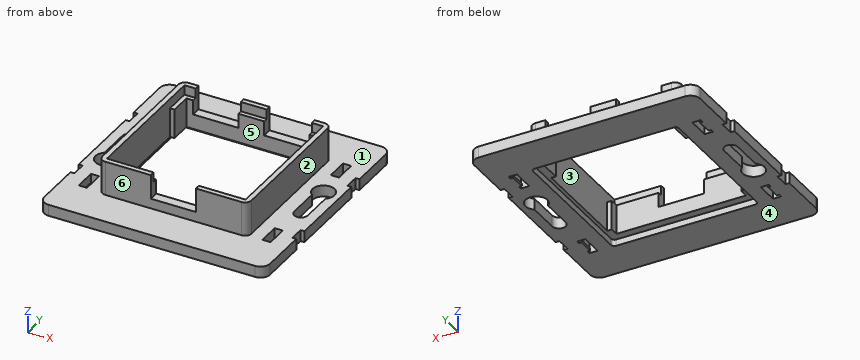
```python
from build123d import *

# Parameters (mm, degrees)
F0_W      = 40.2
F0_H      = 40.2
F1_DEPTH  = 14.1
F2_DEPTH  = 3.5
F3_W      = 1.2
F3_H      = 4.5
F4_DEPTH  = 25
F6_DEPTH  = 2
F7_W      = 43
F7_H      = 43
F7_W_2    = 40.2
F7_H_2    = 40.2
F8_DEPTH  = 3
F9_W      = 14
F9_H      = 7.5
F10_DEPTH = 5
F11_W     = 14
F11_H     = 7.5
F12_DEPTH = 5
F13_W     = 1.4
F13_H     = 31
F14_DEPTH = 15
F15_W     = 0.8
F15_H     = 4.8
F16_DEPTH = 2.7
F17_DEPTH = 7


with BuildPart() as f1:
    # F0 (on Top) → F1 (new body)
    with BuildSketch(Plane.XY):
        with BuildLine():
            Line((23.1, -21.1), (23.1, 21.1))
            ThreePointArc((23.1, 21.1), (22.514214, 22.514214), (21.1, 23.1))
            Line((21.1, 23.1), (-21.1, 23.1))
            ThreePointArc((-21.1, 23.1), (-22.514214, 22.514214), (-23.1, 21.1))
            Line((-23.1, 21.1), (-23.1, -21.1))
            ThreePointArc((-23.1, -21.1), (-22.514214, -22.514214), (-21.1, -23.1))
            Line((-21.1, -23.1), (21.1, -23.1))
            ThreePointArc((21.1, -23.1), (22.514214, -22.514214), (23.1, -21.1))
        make_face()
        Rectangle(F0_W, F0_H, mode=Mode.SUBTRACT)
    extrude(amount=F1_DEPTH)

    # F0 (on Top) → F2 (join)
    with BuildSketch(Plane.XY):
        with BuildLine():
            Line((32, 35), (-32, 35))
            ThreePointArc((-32, 35), (-34.12132, 34.12132), (-35, 32))
            Line((-35, 32), (-35, -32))
            ThreePointArc((-35, -32), (-34.12132, -34.12132), (-32, -35))
            Line((-32, -35), (32, -35))
            ThreePointArc((32, -35), (34.12132, -34.12132), (35, -32))
            Line((35, -32), (35, 32))
            ThreePointArc((35, 32), (34.12132, 34.12132), (32, 35))
        make_face()
        with BuildLine():
            ThreePointArc((21.1, 23.1), (22.514214, 22.514214), (23.1, 21.1))
            Line((23.1, 21.1), (23.1, -21.1))
            ThreePointArc((23.1, -21.1), (22.514214, -22.514214), (21.1, -23.1))
            Line((21.1, -23.1), (-21.1, -23.1))
            ThreePointArc((-21.1, -23.1), (-22.514214, -22.514214), (-23.1, -21.1))
            Line((-23.1, -21.1), (-23.1, 21.1))
            ThreePointArc((-23.1, 21.1), (-22.514214, 22.514214), (-21.1, 23.1))
            Line((-21.1, 23.1), (21.1, 23.1))
        make_face(mode=Mode.SUBTRACT)
    extrude(amount=F2_DEPTH)

    # F3 (on face) → F4 (cut)
    with BuildSketch(Plane.XY.offset(3.5)):
        with Locations((-34.4, 15.25)):
            Rectangle(F3_W, F3_H)
        with Locations((34.4, -15.25)):
            Rectangle(F3_W, F3_H)
        with BuildLine():
            Line((31.85, -5.5), (31.85, 4.326052))
            ThreePointArc((31.85, 4.326052), (29.75, 10.4), (27.65, 4.326052))
            Line((27.65, 4.326052), (27.65, -5.5))
            ThreePointArc((27.65, -5.5), (29.75, -7.6), (31.85, -5.5))
        make_face()
        with BuildLine():
            ThreePointArc((-27.65, 5.5), (-29.75, 7.6), (-31.85, 5.5))
            Line((-31.85, 5.5), (-31.85, -4.326052))
            ThreePointArc((-31.85, -4.326052), (-29.75, -10.4), (-27.65, -4.326052))
            Line((-27.65, -4.326052), (-27.65, 5.5))
        make_face()
        with Locations((34.4, 15.25)):
            Rectangle(F3_W, F3_H)
        with Locations((-34.4, -15.25)):
            Rectangle(F3_W, F3_H)
    extrude(amount=-F4_DEPTH, mode=Mode.SUBTRACT)

    # F5 (on Top) → F6 (cut)
    with BuildSketch(Plane.XY):
        with BuildLine():
            ThreePointArc((-22.6, -21.6), (-22.307107, -22.307107), (-21.6, -22.6))
            Line((-21.6, -22.6), (21.6, -22.6))
            ThreePointArc((21.6, -22.6), (22.307107, -22.307107), (22.6, -21.6))
            Line((22.6, -21.6), (22.6, 21.6))
            ThreePointArc((22.6, 21.6), (22.307107, 22.307107), (21.6, 22.6))
            Line((21.6, 22.6), (-21.6, 22.6))
            ThreePointArc((-21.6, 22.6), (-22.307107, 22.307107), (-22.6, 21.6))
            Line((-22.6, 21.6), (-22.6, -21.6))
        make_face()
    extrude(amount=F6_DEPTH, mode=Mode.SUBTRACT)

    # F7 (on face) → F8 (cut)
    with BuildSketch(Plane.XY.offset(14.1)):
        Rectangle(F7_W, F7_H)
        Rectangle(F7_W_2, F7_H_2, mode=Mode.SUBTRACT)
    extrude(amount=-F8_DEPTH, mode=Mode.SUBTRACT)

    # F9 (on face) → F10 (cut)
    with BuildSketch(Plane.XZ.offset(23.1)):
        with Locations((0, 10.35)):
            Rectangle(F9_W, F9_H)
    extrude(amount=-F10_DEPTH, mode=Mode.SUBTRACT)

    # F11 (on face) → F12 (cut)
    with BuildSketch(Plane(origin=(0, 23.1, 0), x_dir=(-1, 0, 0), z_dir=(0, 1, 0))):
        with Locations((-11, 10.35)):
            Rectangle(F11_W, F11_H)
        with Locations((11, 10.35)):
            Rectangle(F11_W, F11_H)
    extrude(amount=-F12_DEPTH, mode=Mode.SUBTRACT)

    # F13 (on face) → F14 (cut)
    with BuildSketch(Plane.XY.offset(11.1)):
        with Locations((-20.8, -2)):
            Rectangle(F13_W, F13_H)
        with Locations((20.8, -2)):
            Rectangle(F13_W, F13_H)
    extrude(amount=-F14_DEPTH, mode=Mode.SUBTRACT)

    # F15 (on face) → F16 (cut)
    with BuildSketch(Plane.XY.offset(3.5)):
        Polygon((-27.2, 15.55), (-27.2, 22.35), (-29.75, 22.35), (-29.75, 21.35), (-28.95, 21.35), (-28.95, 16.55), (-29.75, 16.55), (-29.75, 15.55), align=None)
        with Locations((-29.35, 18.95)):
            Rectangle(F15_W, F15_H)
        with Locations((29.35, 18.95)):
            Rectangle(F15_W, F15_H)
        Polygon((29.75, 22.35), (27.2, 22.35), (27.2, 15.55), (29.75, 15.55), (29.75, 16.55), (28.95, 16.55), (28.95, 21.35), (29.75, 21.35), align=None)
        Polygon((27.2, -15.55), (27.2, -22.35), (29.75, -22.35), (29.75, -21.35), (28.95, -21.35), (28.95, -16.55), (29.75, -16.55), (29.75, -15.55), align=None)
        with Locations((29.35, -18.95)):
            Rectangle(F15_W, F15_H)
        Polygon((-27.2, -22.35), (-27.2, -15.55), (-29.75, -15.55), (-29.75, -16.55), (-28.95, -16.55), (-28.95, -21.35), (-29.75, -21.35), (-29.75, -22.35), align=None)
        with Locations((-29.35, -18.95)):
            Rectangle(F15_W, F15_H)
    extrude(amount=-F16_DEPTH, mode=Mode.SUBTRACT)

    # F15 (on face) → F17 (cut)
    with BuildSketch(Plane.XY.offset(3.5)):
        Polygon((-27.2, 15.55), (-27.2, 22.35), (-29.75, 22.35), (-29.75, 21.35), (-28.95, 21.35), (-28.95, 16.55), (-29.75, 16.55), (-29.75, 15.55), align=None)
        Polygon((29.75, 22.35), (27.2, 22.35), (27.2, 15.55), (29.75, 15.55), (29.75, 16.55), (28.95, 16.55), (28.95, 21.35), (29.75, 21.35), align=None)
        Polygon((27.2, -15.55), (27.2, -22.35), (29.75, -22.35), (29.75, -21.35), (28.95, -21.35), (28.95, -16.55), (29.75, -16.55), (29.75, -15.55), align=None)
        Polygon((-27.2, -22.35), (-27.2, -15.55), (-29.75, -15.55), (-29.75, -16.55), (-28.95, -16.55), (-28.95, -21.35), (-29.75, -21.35), (-29.75, -22.35), align=None)
    extrude(amount=-F17_DEPTH, mode=Mode.SUBTRACT)


solid = f1.part
```
The model under review builds one solid part; all positions refer to its coordinate system, in mm. Face numbers are marked on the shaded views. A direction names the side the tool comes from. Coordinates: 2 decimals unless noted, no trailing zeros. Write each loop counter-clockwise with the first axis right and the second up, starting at its lowest first coordinate (ties: lowest second). Pieces come first, ordered by that corner, then holes.
1) The part is to be moulded in two halves that separate along X. For the marked faces 1, 2 and 3, say which applies: pulls with the +X half, pulls with the -X half, needs draft (parallel to the pull), parting line crosses it, or undercut.
2) To check wall thickness, follow probe 1 along X at (y, z) = (-2.5, 5); probe 2 along X at (y, z) = (-7, 0.7); probe 3 along X at (y, z) = (12, 2.75). State the ranges of each line that lie inside material, in increasing order.
3) We need section A-A on x = 0. State the section outline as (y, z) points.
4) Machinability: for the marked faces 4, 5 and 6, which of the approach directions +Z, -Z, +X, -X, +Y, -Y give a long, thin tool a straight path to every point of the face, cutting with its end or side? Answer none if there is none.
5) Clearance check with flat-ended pins moving along their axes: pin 1 Ø3 at (x, z) = (-0.5, 8.5) entering from -Y; pin 2 Ø3.5 at (x, y) = (9.5, 22.5) entering from +Z; pin 3 Ø3.5 at (y, z) = (-4, 10) entering from -X. State where each tip first meets the part, or that it passes through.
6) We need section B-B on y = -27.5. State the section outline as (x, z) points.
Answer list:
1. face 1: needs draft
1. face 2: pulls with the +X half
1. face 3: undercut
2. probe 1: x = -23.1 to -21.5, 21.5 to 23.1
2. probe 2: x = -35 to -33.15, -26.35 to -22.6, 22.6 to 28.28, 31.22 to 35
2. probe 3: x = -35 to -21.5, 21.5 to 35
3. outline: (-35, 0) - (-22.6, 0) - (-22.6, 2) - (-20.1, 2) - (-20.1, 6.6) - (-23.1, 6.6) - (-23.1, 3.5) - (-35, 3.5) - close; (20.1, 2) - (22.6, 2) - (22.6, 0) - (35, 0) - (35, 3.5) - (23.1, 3.5) - (23.1, 14.1) - (21.5, 14.1) - (21.5, 11.1) - (20.1, 11.1) - close
4. face 4: -Z, +X, -X, +Y, -Y
4. face 5: +Z, -Z
4. face 6: +Z, +X, -X, -Y
5. pin 1: stops at y = 20.1
5. pin 2: stops at z = 6.6
5. pin 3: stops at x = -23.1
6. outline: (-35, 0) - (35, 0) - (35, 3.5) - (-35, 3.5) - close
